Build history of the part. All positions in model axes, mm. Round coordinates to 2 decimals unless told otherwise and drop trailing zeros. Write each loop counter-clockwise with the first axis right and the second up, starting at its lowest first coordinate (ties: lowest second). Pieces come first, ordered by that corner, then holes. Notation, with made-up numbers: M 41,35 L 59,35 A23 ccw 59,67 Z; hole C 80.5,-38 d10. An arc over 180 degrees is marked long. One line per item, written item: value. Start each with the question number.
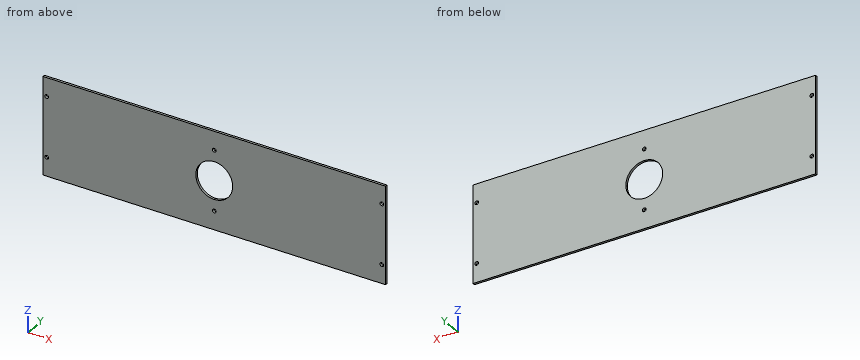
```python
from build123d import *

# Parameters (mm, degrees)
SKETCH1_W           = 372
SKETCH1_H           = 104.22
BOSS_EXTRUDE1_DEPTH = 2.5
SKETCH2_R           = 2
CUT_EXTRUDE1_DEPTH  = 10
SKETCH3_R           = 2
CUT_EXTRUDE2_DEPTH  = 10
CUT_EXTRUDE3_DEPTH  = 26


with BuildPart() as part:
    # Sketch1 → Boss-Extrude1 (new body)
    with BuildSketch(Plane(origin=(0, 0, 0), x_dir=(1, 0, 0), z_dir=(0, 1, 0))):
        with Locations((72.169818201, 7.186191072)):
            Rectangle(SKETCH1_W, SKETCH1_H)
    extrude(amount=BOSS_EXTRUDE1_DEPTH)

    # Sketch2 → Cut-Extrude1 (cut)
    with BuildSketch(Plane(origin=(0, 2.5, 0), x_dir=(1, 0, 0), z_dir=(0, 1, 0))):
        with BuildLine():
            ThreePointArc((-107.830181799, 39.296191072), (-108.415968237, 40.710404634), (-109.830181799, 41.296191072))
            Line((-109.830181799, 41.296191072), (-109.830181799, 39.296191072))
            Line((-109.830181799, 39.296191072), (-111.830181799, 39.296191072))
            ThreePointArc((-111.830181799, 39.296191072), (-109.830181799, 37.296191072), (-107.830181799, 39.296191072))
        make_face()
        with BuildLine():
            Line((-109.830181799, 39.296191072), (-109.830181799, 41.296191072))
            ThreePointArc((-109.830181799, 41.296191072), (-111.244395361, 40.710404634), (-111.830181799, 39.296191072))
            Line((-111.830181799, 39.296191072), (-109.830181799, 39.296191072))
        make_face()
        with BuildLine():
            ThreePointArc((256.169818201, 39.296191072), (255.584031763, 40.710404634), (254.169818201, 41.296191072))
            Line((254.169818201, 41.296191072), (254.169818201, 39.296191072))
            Line((254.169818201, 39.296191072), (256.169818201, 39.296191072))
        make_face()
        with BuildLine():
            Line((254.169818201, 39.296191072), (254.169818201, 41.296191072))
            ThreePointArc((254.169818201, 41.296191072), (252.755604639, 37.88197751), (256.169818201, 39.296191072))
            Line((256.169818201, 39.296191072), (254.169818201, 39.296191072))
        make_face()
        with Locations(Location((-109.830181799, -24.923808928, 0), (0, 0, 270))):
            Circle(SKETCH2_R)
        with Locations(Location((254.169818201, -24.923808928, 0), (0, 0, 270))):
            Circle(SKETCH2_R)
    extrude(amount=-CUT_EXTRUDE1_DEPTH, mode=Mode.SUBTRACT)

    # Sketch3 → Cut-Extrude2 (cut)
    with BuildSketch(Plane(origin=(0, 2.5, 0), x_dir=(1, 0, 0), z_dir=(0, 1, 0))):
        with Locations(Location((72.169818201, 39.296191072, 0), (0, 0, 270))):
            Circle(SKETCH3_R)
        with Locations(Location((72.169818201, -24.923808928, 0), (0, 0, 270))):
            Circle(SKETCH3_R)
    extrude(amount=-CUT_EXTRUDE2_DEPTH, mode=Mode.SUBTRACT)

    # Sketch4 → Cut-Extrude3 (cut)
    with BuildSketch(Plane(origin=(0, 2.5, 0), x_dir=(1, 0, 0), z_dir=(0, 1, 0))):
        with BuildLine():
            ThreePointArc((92.169818201, 7.186191072), (86.311953825, 21.328326696), (72.169818201, 27.186191072))
            Line((72.169818201, 27.186191072), (72.169818201, -12.813808928))
            ThreePointArc((72.169818201, -12.813808928), (86.311953825, -6.955944552), (92.169818201, 7.186191072))
        make_face()
        with BuildLine():
            Line((72.169818201, -12.813808928), (72.169818201, 27.186191072))
            ThreePointArc((72.169818201, 27.186191072), (52.169818201, 7.186191072), (72.169818201, -12.813808928))
        make_face()
    extrude(amount=-CUT_EXTRUDE3_DEPTH, mode=Mode.SUBTRACT)


solid = part.part
```
Item 1: Drill centre lines: line 1 (Z direction, x = 70.5, y = 1.55); line 2 (Z direction, x = 77, y = 0.8); line 3 (X direction, y = 1.8, z = -38). Where is each one in solid material? Low to high.
Item 2: Cut at A-A, the plane y = 2.05. Write the cut outline in (x, z).
Item 3: Cut at B-B, the plane z = -3. Write the cut outline in (x, y), plus the area to 3 significant figures.
Item 4: Cut at C-C, the plane z = -21. Write the cut outline in (x, y).
Computed values:
1. line 1: z = -59.3 to -40.4, -38.2 to -27.12, 12.74 to 23.82, 26.02 to 44.92
1. line 2: z = -59.3 to -26.59, 12.22 to 44.92
1. line 3: x = -113.83 to -111.35, -108.31 to 70.65, 73.69 to 252.65, 255.69 to 258.17
2. outline: M -113.83,-59.3 L 258.17,-59.3 L 258.17,44.92 L -113.83,44.92 Z; hole C -109.83,-39.3 d4; hole C -109.83,24.92 d4; hole C 72.17,-7.19 d40; hole C 72.17,-39.3 d4; hole C 72.17,24.92 d4; hole C 254.17,-39.3 d4; hole C 254.17,24.92 d4
3. outline: M -113.83,0 L 52.61,0 L 52.61,2.5 L -113.83,2.5 Z; M 91.73,0 L 258.17,0 L 258.17,2.5 L 91.73,2.5 Z
3. area: 832 mm2
4. outline: M -113.83,0 L 57.71,0 L 57.71,2.5 L -113.83,2.5 Z; M 86.63,0 L 258.17,0 L 258.17,2.5 L 86.63,2.5 Z
